Read the model definition and answer for the solid it produces. Units are mm, in the model's axes. A direction names the side the tool comes from. Round coordinates to 2 decimals unless told otherwise and drop trailing zeros. Put each result on its own line as item: value.
from build123d import *

# Parameters (mm, degrees)
SKETCH1_W                     = 65
SKETCH1_H                     = 105
BOSS_EXTRUDE1_DEPTH           = 15
BOSS_EXTRUDE1_TAPER           = 1
BOSS_EXTRUDE1_OTHER_WAY_DEPTH = 10
BOSS_EXTRUDE1_OTHER_WAY_TAPER = 1
FILLET1_R                     = 3
BOSS_EXTRUDE2_DEPTH           = 3
BOSS_EXTRUDE2_DEPTH_BACK      = 3
BOSS_EXTRUDE2_START           = 52.5
SKETCH3_W                     = 9.357586106
SKETCH3_H                     = 6.356143016
SKETCH5_R                     = 0.5
CUT_EXTRUDE1_DEPTH            = 3


with BuildPart() as part:
    # Sketch1 → Boss-Extrude1 (new body)
    with BuildSketch(Plane(origin=(0, 0, 0), x_dir=(1, 0, 0), z_dir=(0, 1, 0))):
        Rectangle(SKETCH1_W, SKETCH1_H)
    extrude(amount=BOSS_EXTRUDE1_DEPTH, taper=BOSS_EXTRUDE1_TAPER)

    # Sketch1 → Boss-Extrude1 other way (add)
    with BuildSketch(Plane(origin=(0, 0, 0), x_dir=(1, 0, 0), z_dir=(0, 1, 0))):
        Rectangle(SKETCH1_W, SKETCH1_H)
    extrude(amount=-BOSS_EXTRUDE1_OTHER_WAY_DEPTH, taper=BOSS_EXTRUDE1_OTHER_WAY_TAPER)

    # Fillet1
    fillet1_edges = [part.edges().sort_by_distance(p)[0] for p in [
        (-32.325449351, -10, 0),
        (0, -10, 52.325449351),
        (32.369087013, 7.5, 52.369087013),
        (32.369087013, 7.5, -52.369087013),
        (-32.369087013, 7.5, -52.369087013),
        (-32.369087013, 7.5, 52.369087013),
        (32.238174026, 15, 0),
        (0, 15, -52.238174026),
        (-32.238174026, 15, 0),
        (0, 15, 52.238174026),
        (32.325449351, -10, 0),
        (0, -10, -52.325449351),
        (32.412724675, -5, 52.412724675),
        (-32.412724675, -5, 52.412724675),
        (-32.412724675, -5, -52.412724675),
        (32.412724675, -5, -52.412724675),
    ]]
    fillet(fillet1_edges, radius=FILLET1_R)

    # Sketch3 → Boss-Extrude2 (add, two sides: drawn at the far end of the back side and taken through both)
    with BuildSketch(Plane.XY.offset(BOSS_EXTRUDE2_START - BOSS_EXTRUDE2_DEPTH_BACK)):
        with Locations((20.097339375, 2.5)):
            Rectangle(SKETCH3_W, SKETCH3_H)
    extrude(amount=BOSS_EXTRUDE2_DEPTH + BOSS_EXTRUDE2_DEPTH_BACK)

    # Sketch5 → Cut-Extrude1 (cut)
    with BuildSketch(Plane(origin=(0, 15, 0), x_dir=(1, 0, 0), z_dir=(0, 1, 0))):
        with Locations(Location((19.290082237, -37.5, 0), (0, 0, 270))):
            Circle(SKETCH5_R)
        with Locations(Location((9.290082237, -37.5, 0), (0, 0, 270))):
            Circle(SKETCH5_R)
        with Locations(Location((-0.709917763, -37.5, 0), (0, 0, 270))):
            Circle(SKETCH5_R)
        with Locations(Location((-10.709917763, -37.5, 0), (0, 0, 270))):
            Circle(SKETCH5_R)
        with Locations(Location((-20.709917763, -37.5, 0), (0, 0, 270))):
            Circle(SKETCH5_R)
    extrude(amount=-CUT_EXTRUDE1_DEPTH, mode=Mode.SUBTRACT)


solid = part.part
Item 1: Flat-ended cylindrical pins translate along their axes: pin 1 Ø0.5 at (x, z) = (-21, 37.5) entering from +Y; pin 2 Ø5 at (x, y) = (0, -6.5) entering from -Z; pin 3 Ø8 at (y, z) = (9.5, -35) entering from -X; pin 4 Ø6 at (y, z) = (8, 14) entering from +X. Find the tip coordinate at first contact, or state that the pin passes through.
Derived:
pin 1: stops at y = 15
pin 2: stops at z = -52.43
pin 3: stops at x = -32.4
pin 4: stops at x = 32.41
Item 2: Find the intervals of material crossed by line 1 along X through (y, z) = (12.95, 37.5); line 2 along X through (y, z) = (12.7, 37.5); line 3 along Z through (x, y) = (15, -0.5), in increasing order.
Derived:
line 1: x = -32.14 to -21.21, -20.21 to -11.21, -10.21 to -1.21, -0.21 to 8.79, 9.79 to 18.79, 19.79 to 32.14
line 2: x = -32.21 to -21.21, -20.21 to -11.21, -10.21 to -1.21, -0.21 to 8.79, 9.79 to 18.79, 19.79 to 32.21
line 3: z = -52.49 to 52.49
Item 3: Which of the six approach directions +Z, -Z, +X, -X, +Y, -Y give full straight-line access (tool end or side, diameter ignored) to faces 1 (the flat face through (20, 5.678, 54)), 2 (the flat face through (20, 3, 55.5)), 3 (the flat face through (20, -0.678, 54))?
Derived:
face 1: +Z, +X, -X, +Y
face 2: +Z, +X, -X, +Y, -Y
face 3: +Z, +X, -X, -Y
